Geometry: see drawing. Coordinates: mm, zero at the bounding-box minimum. Coordinates: 2 decimals unless noted, no trailing zeros. Loops run counter-clockwise (first coordinate to the right, second up) from the corner with the lowest first, then second, coordinate; pieces in that order, holes last. Notation, with made-up numbers: (46, 31) - (60, 31) arc R24 ccw to (60, 46) - close; hole circle Ø8 at (40, 58). An arc over 180 degrees is marked (long way). Use a Markdown table: item, result. Add a question column.
1. Section query B-B on y = 38. Return the cut outline in (x, z) (1 decimal).
2. Contact query for flat-ended pins moving along their axis: P1, Ø1.4, axis at x = 2, y = 24.5, coming from the +Z side; P2, Ø4, axis at x = 289.5, y = 25, coming from the -Z side (1 decimal); P3, Ø1.5, axis at y = 7, z = 1, coming from the +X side. Output: stop coordinate, or through.
3. Ray query, L1, parallel to X at y = 30.5, z = 9.25 (1 decimal); L2, parallel to Y at x = 126.5, z = 6; L3, parallel to Z at x = 31, y = 43.5. Return the intervals inside material, ascending. Write a range as [from, to].
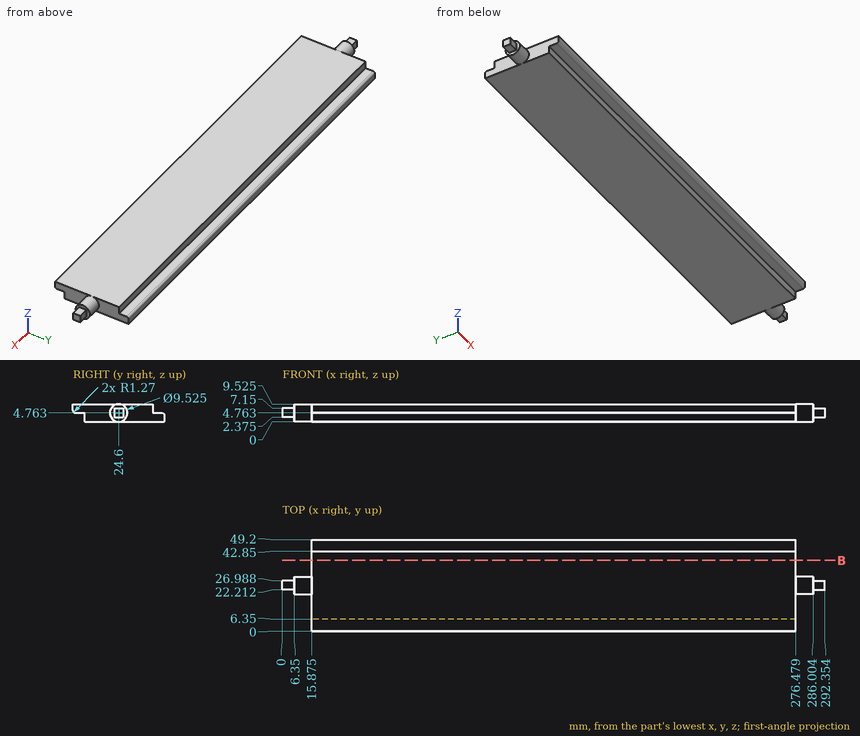
Resolved:
| question | item | result |
|---|---|---|
| 1 | outline | (15.9, 0) - (276.5, 0) - (276.5, 9.5) - (15.9, 9.5) - close |
| 2 | P1 | z = 7.15 |
| 2 | P2 | z = 2.4 |
| 2 | P3 | x = 276.48 |
| 3 | L1 | [15.9, 276.5] |
| 3 | L2 | [0, 42.85] |
| 3 | L3 | [0, 4.76] |
